Geometry check sheet. Reference: the model listing, model coordinates, mm. Face numbers are marked on the shaded views. A direction names the side the tool comes from. Round coordinates to 2 decimals unless told otherwise and drop trailing zeros. Write each loop counter-clockwise with the first axis right and the second up, starting at its lowest first coordinate (ties: lowest second). Pieces come first, ordered by that corner, then holes. Notation, with made-up numbers: (71, -18.75) -> (122, -18.75) arc R25 ccw to (122, 0.25) -> close; hole circle Ø8 at (11.25, -14). An arc over 180 degrees is marked (long way). One line per question, with ' | ' between items.
```python
from build123d import *

# Parameters (mm, degrees)
BOSS_EXTRUDE1_DEPTH = 10
SKETCH2_R           = 1.75
CUT_EXTRUDE1_DEPTH  = 30
SKETCH3_R           = 2.4
CUT_EXTRUDE2_DEPTH  = 15.5
FILLET2_R           = 4
FILLET3_R           = 4
SKETCH5_W           = 9
SKETCH5_H           = 2.25
CUT_EXTRUDE3_DEPTH  = 33
FILLET4_R           = 4
FILLET5_R           = 1


with BuildPart() as part:
    # Sketch1 → Boss-Extrude1 (new body)
    with BuildSketch(Plane(origin=(0, 0, 0), x_dir=(1, 0, 0), z_dir=(0, 1, 0))):
        Polygon((17.5, -2.706437242), (27.5, -2.706437242), (27.5, 6.293562758), (37.5, 6.293562758), (37.5, 11.293562758), (-10, 11.293562758), (-10, 6.293562758), (0, 6.293562758), (0, 0), (0, -2.706437242), (10, -2.706437242), (10, 3.793562758), (17.5, 3.793562758), align=None)
    extrude(amount=BOSS_EXTRUDE1_DEPTH)

    # Sketch2 → Cut-Extrude1 (cut, symmetric)
    with BuildSketch(Plane.ZY.offset(-17.5)):
        with Locations((-0.293562758, 5.096871602)):
            Circle(SKETCH2_R)
    extrude(amount=CUT_EXTRUDE1_DEPTH, both=True, mode=Mode.SUBTRACT)

    # Sketch3 → Cut-Extrude2 (cut, symmetric)
    with BuildSketch(Plane.XY.offset(-6.293562758)):
        with Locations(Location((-5, 5, 0), (0, 0, 180))):
            Circle(SKETCH3_R)
        with Locations(Location((32.5, 5, 0), (0, 0, 180))):
            Circle(SKETCH3_R)
    extrude(amount=CUT_EXTRUDE2_DEPTH, both=True, mode=Mode.SUBTRACT)

    # Fillet2
    fillet2_edges = [part.edges().sort_by_distance(p)[0] for p in [
        (22.5, 0, 2.706437242),
        (5, 0, 2.706437242),
    ]]
    fillet(fillet2_edges, radius=FILLET2_R)

    # Fillet3
    fillet3_edges = [part.edges().sort_by_distance(p)[0] for p in [
        (37.5, 10, -8.793562758),
        (-10, 0, -8.793562758),
        (37.5, 0, -8.793562758),
        (-10, 10, -8.793562758),
    ]]
    fillet(fillet3_edges, radius=FILLET3_R)

    # Sketch5 → Cut-Extrude3 (cut, symmetric)
    with BuildSketch(Plane(origin=(27.5, 0, 0), x_dir=(0, 0, -1), z_dir=(1, 0, 0))):
        with Locations((1.793562758, 8.875)):
            Rectangle(SKETCH5_W, SKETCH5_H)
    extrude(amount=CUT_EXTRUDE3_DEPTH, both=True, mode=Mode.SUBTRACT)

    # Fillet4
    # the kernel refuses this fillet: 4 mm, written as the material it takes off along each edge
    with BuildSketch(Plane(origin=(7.519550361, 7.75, 2.706437242), x_dir=(0, 0, -1), z_dir=(1, 0, 0))) as fillet4_piece_1:
        with BuildLine():
            CenterArc((3.992179856, -4), FILLET4_R, 90, 86.416678302)
            Line((0, -3.75), (-0.079843597, -3.745))
            ThreePointArc((-0.079843597, -3.745), (-0.08, -1.875), (-0.08, 0))
            Line((-0.08, 0), (0, 0.08))
            Line((0, 0.08), (3.992179856, 0.08))
            Line((3.992179856, 0.08), (3.992179856, 0))
        make_face()
    extrude(amount=29.960899278, mode=Mode.SUBTRACT)
    with BuildSketch(Plane(origin=(-9.980449639, 7.75, 2.706437242), x_dir=(0, -1, 0), z_dir=(1, 0, 0))) as fillet4_piece_2:
        with BuildLine():
            CenterArc((4, 3.992179856), FILLET4_R, 180, 86.416678302)
            Line((0, 3.992179856), (-0.08, 3.992179856))
            Line((-0.08, 3.992179856), (-0.08, 0))
            Line((-0.08, 0), (0, -0.08))
            ThreePointArc((0, -0.08), (1.875, -0.08), (3.745, -0.079843597))
            Line((3.745, -0.079843597), (3.75, 0))
        make_face()
    extrude(amount=29.960899278, mode=Mode.SUBTRACT)

    # Fillet5
    fillet5_edges = [part.edges().sort_by_distance(p)[0] for p in [
        (27.5, 3.875, -6.293562758),
        (0, 3.875, -6.293562758),
        (13.75, 7.75, -6.293562758),
    ]]
    fillet(fillet5_edges, radius=FILLET5_R)


solid = part.part
```
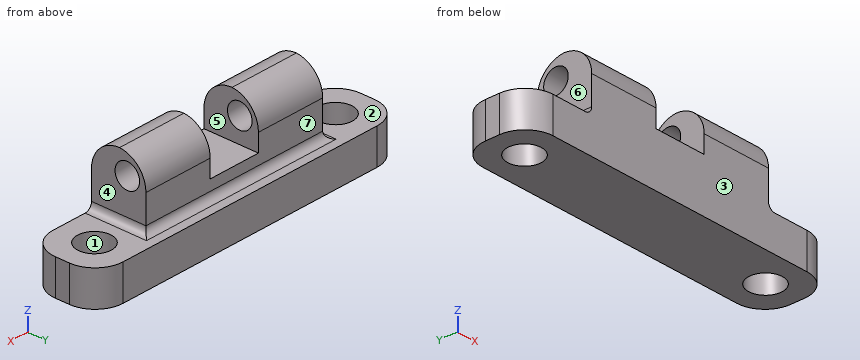
(1) Material ranges on line 1 (X direction, y = 5, z = -8.8); line 2 (Y direction, x = 17.5, z = -4); line 3 (Y direction, x = 32.5, z = -9.1), recorded low to high.
Resolved:
line 1: x = -10 to -7.4, -2.6 to 30.1, 34.9 to 37.5 | line 2: y = 0 to 7.75 | line 3: y = 0 to 2.6, 7.4 to 10
(2) Go/stop test with flat-tipped pins: pin 1 (5.5 mm diameter, centred on x = 32.5, y = 5, fed in from +Z); pin 2 (2 mm diameter, centred on y = 4.5, z = -2, fed in from -X); pin 3 (4.5 mm diameter, centred on x = 17.5, z = -2.5, fed in from +Y). Record where each tip stops, or that it passes through.
Resolved:
pin 1: stops at z = -6.29 | pin 2: stops at x = 0 | pin 3: stops at y = 7.75
(3) Sectioned sample at D-D on y = 2. Record the cut outline in (x, z).
Resolved:
outline: (-9.46, -11.29) -> (36.96, -11.29) -> (36.96, -6.29) -> (28.5, -6.29) arc R1 cw to (27.5, -5.29) -> (27.5, 2.17) -> (17.5, 2.17) -> (17.5, -3.79) -> (10, -3.79) -> (10, 2.17) -> (0, 2.17) -> (0, -5.29) arc R1 cw to (-1, -6.29) -> (-9.46, -6.29) -> close
(4) Access from +Z, -Z, +X, -X, +Y, -Y to the whole of each face (thin tool, end or side, straight path). Record for the marked faces 4, 5, 6 and 7.
Resolved:
face 4: +Z, +X, +Y, -Y | face 5: +Z, +Y, -Y | face 6: +Z, -X, +Y, -Y | face 7: +Z, +X, -X, +Y
(5) Sectioned sample at A-A on x = -5. Record the cut outline in (y, z).
Resolved:
outline: (0, -11.29) -> (2.6, -11.29) -> (2.6, -6.29) -> (0, -6.29) -> close; (7.4, -11.29) -> (10, -11.29) -> (10, -6.29) -> (7.4, -6.29) -> close
(6) Draft check along Y on the marked faces 1, 2 and 3. Enter one of: +Y half, -Y half, draft (parallel to the pull), parting line (faces both ways), or undercut.
Resolved:
face 1: undercut | face 2: draft | face 3: -Y half
(7) Sectioned sample at C-C on x = 15. Record the cut outline in (y, z).
Resolved:
outline: (0, -11.29) -> (10, -11.29) -> (10, -6.29) -> (8.75, -6.29) arc R1 cw to (7.75, -5.29) -> (7.75, -3.79) -> (0, -3.79) -> close
(8) Sectioned sample at B-B on z = -0.5. Record the cut outline in (x, y).
Resolved:
outline: (0, 0.08) -> (10, 0.08) -> (10, 3.36) -> (0, 3.36) -> close; (0, 6.83) -> (10, 6.83) -> (10, 7.67) -> (0, 7.67) -> close; (17.5, 0.08) -> (27.5, 0.08) -> (27.5, 3.36) -> (17.5, 3.36) -> close; (17.5, 6.83) -> (27.5, 6.83) -> (27.5, 7.67) -> (17.5, 7.67) -> close
